Could you check a few things on this drawing? It's one solid part, dimensions in mm from its lowest x, y, z. Give positions to 0.01 mm unless a question says otherwise; leave off trailing zeros. Loops run counter-clockwise (first coordinate to the right, second up) from the corner with the lowest first, then second, coordinate; pieces in that order, holes last. Notation, with made-up numbers: (23, -35) - (52, -35) arc R30 cw to (52, -10) - close; hole circle Ø3 at (-3.5, -16). An arc over 180 degrees is marked (long way). Return JSON: item names as keys, results as strings. Group by question number.
(1) If we section it at B-B (z = 4.25): Please give me the cut outline in (x, y).
(2) If we section it at C-C (x = 3): Please give me the cut outline in (y, z).
(3) If we section it at D-D (x = 25): Please give me the cut outline in (y, z).
(4) I need wall thicknesses on probe 1 along X at (y, z) = (12.5, 6.5); probe 2 along X at (y, z) = (9.5, 7.5); probe 3 along Z at (x, y) = (63.5, 13.25). Which ranges of each line are inside material? Lowest first, please. Write a range as [from, to].
(5) If we mould it in two halves opening along X, with no side actions, what happens to the marked faces 1 and 2? For each: released by +X, released by -X, zero draft, split by the parting line, or undercut.
(6) If we section it at A-A (y = 6.75): Please give me the cut outline in (x, z), then the cut area to 3 significant figures.
(7) For P1, Ø5, axis at x = 79.5, y = 6.5, coming from the -Z side; P2, Ø4.5, axis at x = 31, y = 7, coming from the -Z side; P3, Ø1.6, axis at y = 11, z = 7, coming from the +X side, each with a flat end and sliding along its axis, tell me the tip position at first contact or that it passes through.
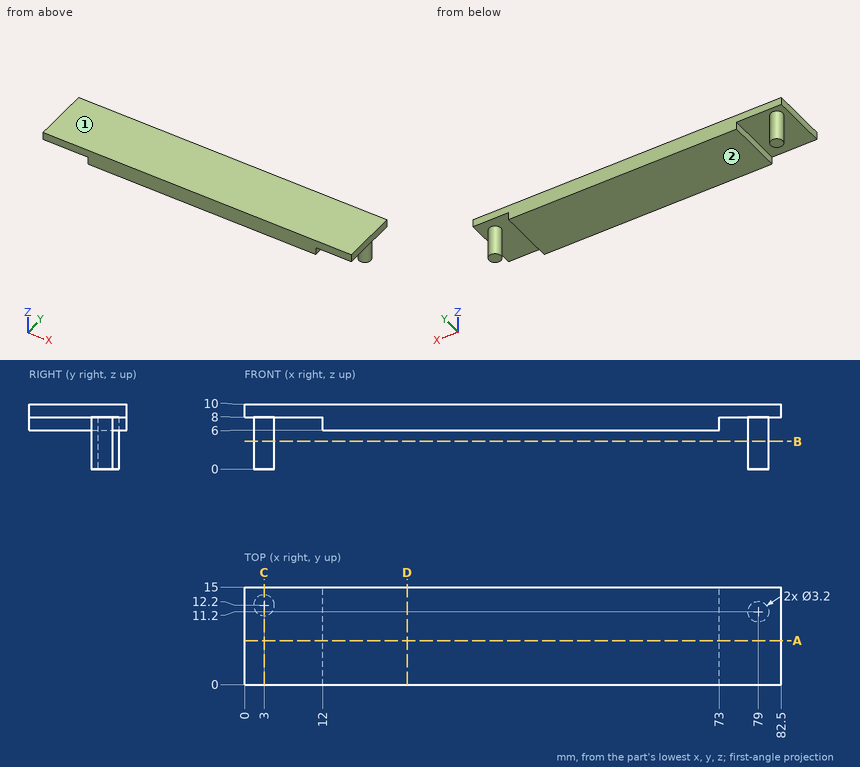
Values:
{
 "1": {"outline": "circle Ø3.2 at (3, 12.2); circle Ø3.2 at (79, 11.2)"},
 "2": {"outline": "(0, 8) - (10.6, 8) - (10.6, 0) - (13.8, 0) - (13.8, 8) - (15, 8) - (15, 10) - (0, 10) - close"},
 "3": {"outline": "(0, 6) - (15, 6) - (15, 10) - (0, 10) - close"},
 "4": {"probe 1": "[1.43, 4.57], [12, 73], [78.07, 79.93]", "probe 2": "[12, 73]", "probe 3": "[6, 10]"},
 "5": {"face 1": "zero draft", "face 2": "undercut"},
 "6": {"outline": "(0, 8) - (12, 8) - (12, 6) - (73, 6) - (73, 8) - (82.5, 8) - (82.5, 10) - (0, 10) - close", "area": "287 mm2"},
 "7": {"P1": "z = 8", "P2": "z = 6", "P3": "x = 80.6"}
}
